from build123d import *

# Parameters (mm, degrees)
EXTRUDE_1_DEPTH     = 2
SKETCH_3_R          = 4
SKETCH_3_R_2        = 1.5
EXTRUDE_2_DEPTH     = 4
SKETCH_3_3_R        = 4
EXTRUDE_3_DEPTH     = 0.4
FILLET_1_R          = 2
SKETCH_3_4_R        = 1.5
CUT_EXTRUDE_1_DEPTH = 5


with BuildPart() as part:
    # Sketch 2 → Extrude 1 (new, symmetric)
    with BuildSketch(Plane.XY):
        with BuildLine():
            Line((6, 40), (6, -40))
            ThreePointArc((6, -40), (0, -46), (-6, -40))
            Line((-6, -40), (-6, 40))
            ThreePointArc((-6, 40), (0, 46), (6, 40))
        make_face()
    extrude(amount=EXTRUDE_1_DEPTH, both=True)

    # Sketch 3 → Extrude 2 (add)
    # profile 1 of 3: a face of its own
    with BuildSketch(Plane(origin=(0, 0, -2), x_dir=(-1, 0, 0), z_dir=(0, 0, -1))):
        with Locations(Location((0, 40, 0), (0, 0, 180))):
            Circle(SKETCH_3_R)
        with Locations((0, 40)):
            Circle(SKETCH_3_R_2, mode=Mode.SUBTRACT)
    # profile 2 of 3: a face of its own
    with BuildSketch(Plane(origin=(0, 0, -2), x_dir=(-1, 0, 0), z_dir=(0, 0, -1))):
        with Locations(Location((0, 0, 0), (0, 0, 180))):
            Circle(SKETCH_3_R)
        Circle(SKETCH_3_R_2, mode=Mode.SUBTRACT)
    # profile 3 of 3: a face of its own
    with BuildSketch(Plane(origin=(0, 0, -2), x_dir=(-1, 0, 0), z_dir=(0, 0, -1))):
        with Locations(Location((0, -40, 0), (0, 0, 180))):
            Circle(SKETCH_3_R)
        with Locations((0, -40)):
            Circle(SKETCH_3_R_2, mode=Mode.SUBTRACT)
    extrude(amount=EXTRUDE_2_DEPTH)

    # Sketch 3_3 → Extrude 3 (add)
    # profile 1 of 2: a face of its own
    with BuildSketch(Plane(origin=(0, 0, -2), x_dir=(-1, 0, 0), z_dir=(0, 0, -1))):
        with BuildLine():
            ThreePointArc((-6, 40), (0, 34), (6, 40))
            ThreePointArc((6, 40), (0, 46), (-6, 40))
        make_face()
        with Locations((0, 40)):
            Circle(SKETCH_3_3_R, mode=Mode.SUBTRACT)
    # profile 2 of 2: a face of its own
    with BuildSketch(Plane(origin=(0, 0, -2), x_dir=(-1, 0, 0), z_dir=(0, 0, -1))):
        with BuildLine():
            ThreePointArc((-6, -40), (0, -46), (6, -40))
            ThreePointArc((6, -40), (0, -34), (-6, -40))
        make_face()
        with Locations((0, -40)):
            Circle(SKETCH_3_3_R, mode=Mode.SUBTRACT)
    extrude(amount=EXTRUDE_3_DEPTH)

    # Fillet 1
    fillet_1_edges = [part.edges().sort_by_distance(p)[0] for p in [
        (0, -46, 2),
        (6, 0, 2),
        (0, 46, 2),
        (-6, 0, 2),
    ]]
    fillet(fillet_1_edges, radius=FILLET_1_R)

    # Sketch 3_4 → Cut-Extrude 1 (cut, symmetric)
    with BuildSketch(Plane(origin=(0, 0, -2), x_dir=(-1, 0, 0), z_dir=(0, 0, -1))):
        with Locations(Location((0, 40, 0), (0, 0, 180))):
            Circle(SKETCH_3_4_R)
        with Locations(Location((0, 0, 0), (0, 0, 180))):
            Circle(SKETCH_3_4_R)
        with Locations(Location((0, -40, 0), (0, 0, 180))):
            Circle(SKETCH_3_4_R)
    extrude(amount=CUT_EXTRUDE_1_DEPTH, both=True, mode=Mode.SUBTRACT)


solid = part.part
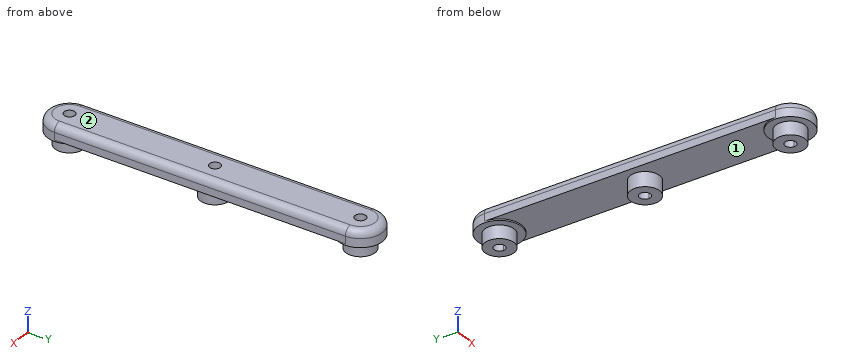
Design review of the part built by this model. Coordinates are the model's own, in mm. Face numbers are marked on the shaded views. Coordinates: 2 decimals unless noted, no trailing zeros. Order: outer loops, then holes, each group sorted by start corner. A loop starts at its lowest first (then second) coordinate and runs counter-clockwise, first axis right, second up. Notation, with made-up numbers: (8.5, 32) - (23.5, 32) arc R33 cw to (23.5, 65) - close; hole circle Ø8 at (-26.5, 33). An arc over 180 degrees is marked (long way). Put each result on its own line as item: value.
1) Take a section at C-C, the plane y = 32. Give the boundary of the cut face in (x, z).
Response values:
outline: (-6, -2) - (6, -2) - (6, 0) arc R2 ccw to (4, 2) - (-4, 2) arc R2 ccw to (-6, 0) - close
2) Insertion check: P1, Ø2.5, axis at x = 0, y = -40, coming from the -Z side; P2, Ø3.5, axis at x = -2, y = -9, coming from the -Z side; P3, Ø4, axis at x = 0, y = 0, coming from the +Z side; P4, Ø3, axis at x = 4.5, z = -5, coming from the -Y side. Each pin has a flat end and moves straight along its axis. Give the tip position at first contact, or say it passes through.
Response values:
P1: passes through
P2: stops at z = -2
P3: stops at z = 2
P4: stops at y = -42.65
3) Wall thickness on L1, parallel to Y at x = 0, z = -0.2; L2, parallel to Y at x = -3.5, z = -5; L3, parallel to Y at x = -0.5, z = -3.5: over which ranges is each line inside the solid? List them lowest first. Write a range as from..to.
Response values:
L1: y = -46..-41.5, -38.5..-1.5, 1.5..38.5, 41.5..46
L2: y = -41.94..-38.06, -1.94..1.94, 38.06..41.94
L3: y = -43.97..-41.41, -38.59..-36.03, -3.97..-1.41, 1.41..3.97, 36.03..38.59, 41.41..43.97
4) Take a section at A-A, the plane x = 0. Count the separate pieces of the cut face and the enclosed holes in it, and give its area (3 significant figures).
Response values:
separate pieces: 4
enclosed holes: 0
area: 393 mm²
5) The part is to be moulded in two halves that separate along Y. For the marked faces 1 and 2, say which applies: released by +Y, released by -Y, zero draft, split by the parting line, or undercut.
Response values:
face 1: undercut
face 2: zero draft
6) Take a section at B-B, the plane z = -1. Give the boundary of the cut face in (x, y), and give its area (3 significant figures).
Response values:
outline: (-6, -40) arc R6 ccw to (6, -40) - (6, 40) arc R6 ccw to (-6, 40) - close; hole circle Ø3 at (0, -40); hole circle Ø3 at (0, 0); hole circle Ø3 at (0, 40)
area: 1,050 mm²
